For this review, take the finished solid that the model builds, in its own axes (mm). Face numbers are marked on the shaded views. A direction names the side the tool comes from. Coordinates: 2 decimals unless noted, no trailing zeros. Write each loop counter-clockwise with the first axis right and the second up, starting at its lowest first coordinate (ties: lowest second). Pieces come first, ordered by that corner, then holes. Notation, with made-up numbers: (1.5, -30.5) -> (39.5, -30.5) arc R22 cw to (39.5, -3.5) -> close; hole circle Ø2 at (36, 62.25). An arc over 180 degrees is marked (long way). Put each result on its own line as item: value. Start each with the question number.
Item 1: Consider section C-C on y = 0. Give the boundary of the cut face in (x, z), and give its area (3 significant figures).
Item 2: Insertion check: P1, Ø1.5, axis at y = -14.5, z = 1, coming from the +X side; P2, Ø1, axis at x = 5.5, z = -8, coming from the -Y side; P3, Ø1, axis at x = -8, z = -5.5, coming from the -Y side. Each pin has a flat end and moves straight along its axis. Give the tip position at first contact, or say it passes through.
Item 3: Consider section D-D on x = -13. Give the boundary of the cut face in (y, z), and give its area (3 significant figures).
Item 4: Consider section A-A on x = 0. Give the boundary of the cut face in (y, z).
Item 5: To check wall thickness, follow L1, parallel to Y at x = 0, z = -2.5; L2, parallel to Y at x = 4.5, z = -3.5; L3, parallel to Z at x = 8, y = 12. State the ranges of each line that lie inside material, in increasing order.
Item 6: Consider section B-B on z = -2.75. Give the boundary of the cut face in (x, y).
Item 7: For the marked faces 1 and 2, list the 3-axis set-ups (+Z, -Z, +X, -X, +Y, -Y) from which the entire face can be reached by the end or side of a thin tool; tool diameter is ignored.
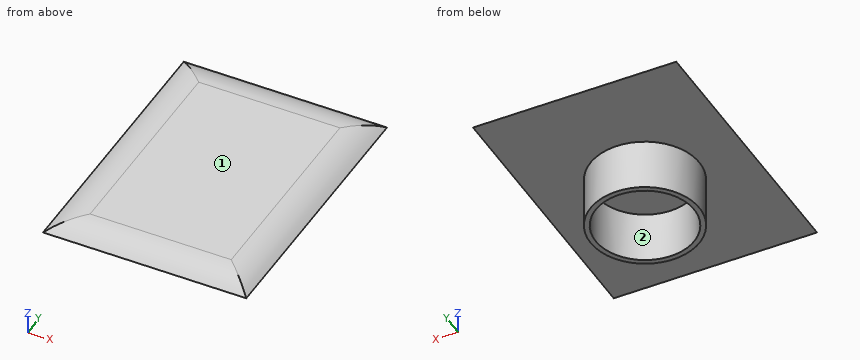
```python
from build123d import *

# Parameters (mm, degrees)
F0_R        = 10.5
F0_R_2      = 9.5
F1_DEPTH    = 10
F2_W        = 39.2694026232
F2_H        = 52.6303946972
F3_DEPTH    = 1
F4_DEPTH    = 1
F5_T1_DEPTH = 82.6303946972
F5_T3_DEPTH = 69.2694026232


# Not quite as in the source:
# - a fillet or chamfer that OpenCascade refuses, or shapes differently, is made with other operations: its cross-section is extruded or revolved along the edge and cut away or added


with BuildPart() as f1:
    # F0 (on Top) → F1 (new body)
    with BuildSketch(Plane.XY):
        Circle(F0_R)
        Circle(F0_R_2, mode=Mode.SUBTRACT)
    extrude(amount=-F1_DEPTH)

    # F2 (on Top) → F3 (join)
    with BuildSketch(Plane.XY):
        Rectangle(F2_W, F2_H)
    extrude(amount=F3_DEPTH)

    # F4 (add): a face of the model
    f4_faces = [f1.faces().sort_by_distance(p)[0] for p in [
        (0, 0, 1),
    ]]
    extrude(f4_faces, amount=F4_DEPTH)

    # F5: fillet of radius 10 on 4 edges, made by hand

    # F5_s2 → F5_t1 (cut)
    with BuildSketch(Plane.XZ.offset(-41.3151973486)):
        with BuildLine():
            ThreePointArc((19.6347013116, 0), (16.7969789718, 1.4868329805), (13.6347013116, 2))
            Line((13.6347013116, 2), (19.6347013116, 2))
            Line((19.6347013116, 2), (19.6347013116, 0))
        make_face()
        with BuildLine():
            ThreePointArc((-19.6347013116, 0), (-16.7969789718, 1.4868329805), (-13.6347013116, 2))
            Line((-13.6347013116, 2), (-19.6347013116, 2))
            Line((-19.6347013116, 2), (-19.6347013116, 0))
        make_face()
    extrude(amount=F5_T1_DEPTH, mode=Mode.SUBTRACT)

    # F5_s4 → F5_t3 (cut)
    with BuildSketch(Plane.YZ.offset(-34.6347013116)):
        with BuildLine():
            ThreePointArc((26.3151973486, 0), (23.4774750088, 1.4868329805), (20.3151973486, 2))
            Line((20.3151973486, 2), (26.3151973486, 2))
            Line((26.3151973486, 2), (26.3151973486, 0))
        make_face()
        with BuildLine():
            ThreePointArc((-20.3151973486, 2), (-23.4774750088, 1.4868329805), (-26.3151973486, 0))
            Line((-26.3151973486, 0), (-26.3151973486, 2))
            Line((-26.3151973486, 2), (-20.3151973486, 2))
        make_face()
    extrude(amount=F5_T3_DEPTH, mode=Mode.SUBTRACT)


solid = f1.part
```
Return value:
1. outline: (-19.63, 0) -> (-10.5, 0) -> (-10.5, -10) -> (-9.5, -10) -> (-9.5, 0) -> (9.5, 0) -> (9.5, -10) -> (10.5, -10) -> (10.5, 0) -> (19.63, 0) arc R10 ccw to (13.63, 2) -> (-13.63, 2) arc R10 ccw to start
1. area: 90.9 mm^2
2. P1: x = 19.29
2. P2: y = -9.23
2. P3: y = -7.35
3. outline: (-26.32, 0) -> (26.32, 0) arc R10 ccw to (20.32, 2) -> (-20.32, 2) arc R10 ccw to start
3. area: 97.6 mm^2
4. outline: (-26.32, 0) -> (-10.5, 0) -> (-10.5, -10) -> (-9.5, -10) -> (-9.5, 0) -> (9.5, 0) -> (9.5, -10) -> (10.5, -10) -> (10.5, 0) -> (26.32, 0) arc R10 ccw to (20.32, 2) -> (-20.32, 2) arc R10 ccw to start
5. L1: -10.5 to -9.5, 9.5 to 10.5
5. L2: -9.49 to -8.37, 8.37 to 9.49
5. L3: 0 to 2
6. outline: circle Ø21 at (0, 0); hole circle Ø19 at (0, 0)
7. face 1: +Z, +X, -X, +Y, -Y
7. face 2: -Z
